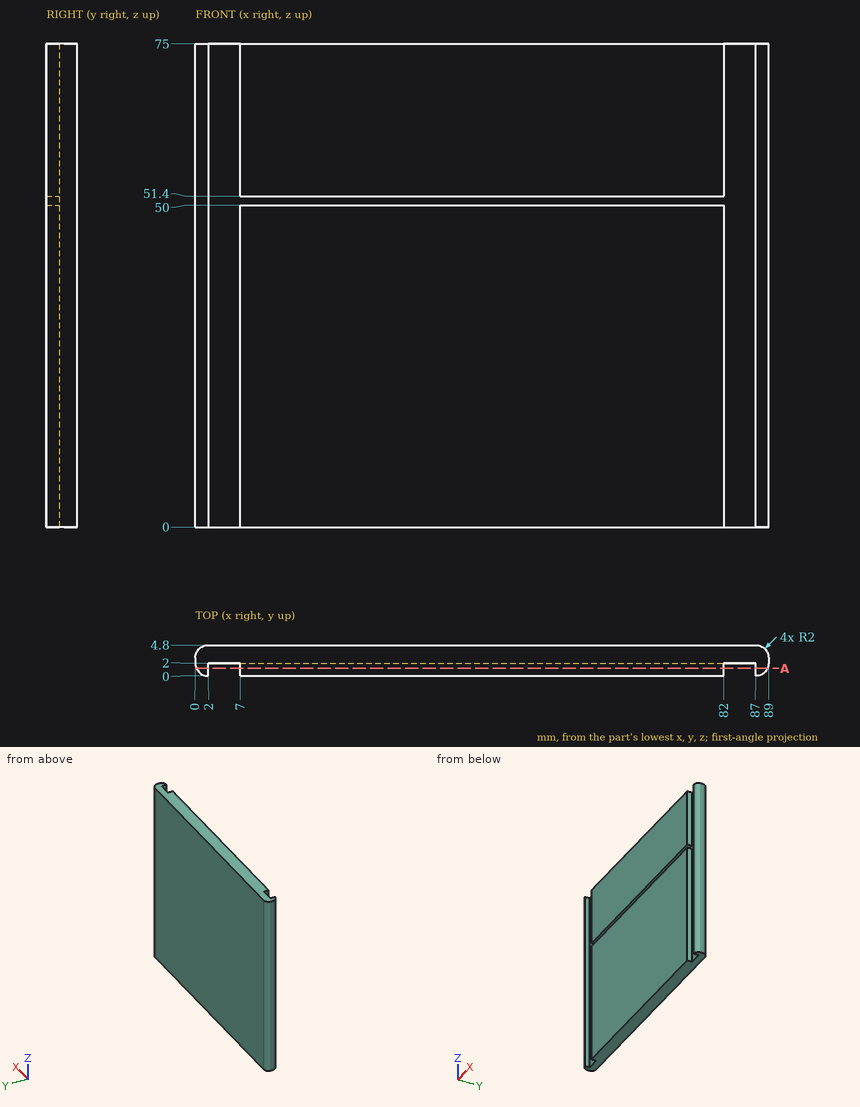
Input: dimensioned drawing with shaded views. Units: mm. Origin: part minimum x, y, z. Coordinates: 2 decimals unless noted, no trailing zeros. Order: outer loops, then holes, each group sorted by start corner. A loop starts at its lowest first (then second) coordinate and runs counter-clockwise, first axis right, second up. Notation, with made-up numbers: (3, 28) -> (39, 28) arc R22 cw to (39, 51) -> close; hole circle Ø3 at (64, -7). An arc over 180 degrees is marked (long way). Use CSV: the item, a comma, the result in double quotes.
1) Line query: line 1 (X direction, y = 1.7, z = 29.5); line 2 (Z direction, x = 75.5, y = 1.35); line 3 (X direction, y = 1.55, z = 66). Output: solid intervals per line, ascending.
Findings:
line 1,"x = 0.02 to 2, 7 to 82, 87 to 88.98"
line 2,"z = 0 to 50, 51.4 to 75"
line 3,"x = 0.05 to 2, 7 to 82, 87 to 88.95"
2) Pin query (flat end, axial travel): pin 1 Ø2 at (y, z) = (1, 47) entering from -X; pin 2 Ø0.6 at (y, z) = (1, 20) entering from +X. Return the tip coordinate at first contact, or that it passes through.
Findings:
pin 1,"stops at x = 0"
pin 2,"stops at x = 88.87"
3) Section A-A on y = 1.2. Output: boundary loops of the cut face in (x, z).
Findings:
outline,"(0.17, 0) -> (2, 0) -> (2, 75) -> (0.17, 75) -> close; (7, 0) -> (82, 0) -> (82, 50) -> (7, 50) -> close; (7, 51.4) -> (82, 51.4) -> (82, 75) -> (7, 75) -> close; (87, 0) -> (88.83, 0) -> (88.83, 75) -> (87, 75) -> close"
